The listing builds one solid part. Answer for the finished solid, in the listing's coordinates (mm). A direction names the side the tool comes from. Coordinates: 2 decimals unless noted, no trailing zeros. Loops run counter-clockwise (first coordinate to the right, second up) from the corner with the lowest first, then second, coordinate; pieces in that order, holes last. Notation, with made-up numbers: M 62.25,71 L 80.25,71 A20 cw 80.25,80 Z; hole C 7,52 d5. An arc over 180 degrees is marked long. Return JSON: item names as keys, results as strings. Group by question number.
1. Straight lines are drawn through the part: L1, parallel to Z at x = 30, y = -10; L2, parallel to X at y = -5.75, z = 19; L3, parallel to X at y = 10.25, z = 1.95. For each, find the intervals that lie inside material, in ascending order. Write a range as from..to.
2. Section C-C (y = 5) is taken. Count the separate pieces of the cut face and the enclosed holes in it, then the cut area to 3 significant figures.
3. Section D-D (x = -19) is taken. Write down the section's boundary in (y, z), then the cut area to 3 significant figures.
4. Given P1, Ø4.5, axis at x = -30, z = 11, coming from the +Y side; P2, Ø1.6, axis at x = -24, z = 11, coming from the +Y side; P3, Ø12, axis at x = -9, y = -14.5, coming from the +Z side, each flat-ended and moving along its own axis, determine where each tip first touches the part or whether it passes through.
5. Section B-B (z = 14.75) is taken. Write down the section's boundary in (x, y), then the cut area to 3 significant figures.
6. The mould has two halves that part along Y. Classify faces 6 (the face through (-10.32, 17.07, 2.54)), 7 (the face through (-22.8, -5.93, 11.62)), 8 (the face through (-27, 6.75, 14)): pulls with the +Y half, pulls with the -Y half, needs draft (parallel to the pull), parting line crosses it, or undercut.
7. Section A-A (y = 10.25) is taken. Write down the section's boundary in (x, z), then the cut area to 4 significant figures.
8. Which of the six approach directions +Z, -Z, +X, -X, +Y, -Y give full straight-line access (tool end or side, diameter ignored) to faces 1 (the face through (-20, -9, 14)), 2 (the face through (11.68, 17.07, 2.54)), 3 (the face through (-28.8, -5.93, 19.62)), 4 (the face through (0, -5, 0)), 5 (the face through (27, 6.75, 14))?
Autodesk Inventor part; units mm, degrees
ref_plane "YZ Plane" through (0, 0, 0) normal (1, 0, 0) x (0, 1, 0)
ref_plane "XZ Plane" through (0, 0, 0) normal (0, 1, 0) x (-1, 0, 0)
ref_plane "XY Plane" through (0, 0, 0) normal (0, 0, 1) x (1, 0, 0)
sketch "Sketch1" plane through (0, 0, 0) normal (0, 0, 1) x (1, 0, 0)
  line L0 (0, 0) -> (36, 0)
  line L1 (36, 0) -> (36, 25)
  line L2 (36, 25) -> (-36, 25)
  line L3 (-36, 25) -> (-36, -25)
  line L4 (-36, -25) -> (36, -25)
  line L5 (36, -25) -> (36, 25)
  dimension "d0" = 36
  dimension "d1" = 25
  dimension "d2" = 72
  dimension "d3" = 50
extrude "Extrusion1" add sketch "Sketch1" along normal blind 5
sketch "Sketch2" plane through (0, 0, 5) normal (0, 0, 1) x (1, 0, 0)
  line L0 (0, 0) -> (0, -25)
  line L1 (-36, -25) -> (36, -25)
  line L2 (0, -25) -> (0, 10.25)
  circle A0 centre (0, 10.25) radius 11.25
  dimension "d6" = 35.25
  dimension "d7" = 22.5
extrude "Extrusion2" cut sketch "Sketch2" against normal blind 22.5
sketch "Sketch3" plane through (0, 0, 5) normal (0, 0, 1) x (1, 0, 0)
  line L0 (0, 0) -> (11, 0)
  line L1 (11, -24.8696) -> (11, -21.6196)
  circle A0 centre (11, -21.6196) radius 1.475
  line L2 (0, 0) -> (0, -3.6992)
  circle A1 centre (-11, -21.6196) radius 1.475
  line L3 (11, -21.6196) -> (11, 18.3804)
  line L4 (11, -21.6196) -> (11, -1.6196)
  line L5 (11, -1.6196) -> (-3.4092, -1.6196)
  circle A2 centre (11, 18.3804) radius 1.475
  circle A3 centre (-11, 18.3804) radius 1.475
  point P0 (0, -1.6196)
  point P1 (11, -20.1446)
  point P2 (11, -23.0946)
  dimension "d10" = 11
  dimension "d11" = 3.25
  dimension "d12" = 2.95
  dimension "d15" = 40
  dimension "d16" = 20
extrude "Extrusion3" cut sketch "Sketch3" against normal blind 5 contours A0 L1 L3 | L3 L1 A0 | A1
sketch "Sketch4" plane through (0, 0, 5) normal (0, 0, 1) x (1, 0, 0)
  point P0 (0, 0)
extrude "Extrusion4" cut sketch "Sketch3" against normal blind 5 contours A2 | A3
sketch "Sketch5" plane through (36, -25, 0) normal (1, 0, 0) x (0, 0, -1)
  line L0 (0, 0) -> (0, 50)
  line L1 (-5, 0) -> (-5, 50)
  line L2 (0, 0) -> (-5, 0)
  line L3 (-5, 0) -> (-5, 50)
  line L4 (-5, 50) -> (0, 50)
  line L5 (0, 50) -> (0, 0)
  point P0 (0, 25)
  dimension "d19" = 5
ref_plane "Work Plane1" through (0, -25, 0) normal (1, 0, 0) x (0, 0, -1)
extrude "Extrusion5" cut sketch "Sketch5" against normal blind 1.5
mirror "Mirror1" about plane through (0, -25, 0) normal (1, 0, 0) of "Extrusion5"
sketch "Sketch6" plane through (34.5, -25, 0) normal (1, 0, 0) x (0, 0, -1)
  line L0 (-5, 0) -> (0, 0)
  line L1 (-5, 0) -> (-23, 0)
  line L2 (-23, 0) -> (-23, 34.75)
  line L3 (-23, 34.75) -> (-5, 34.75)
  line L4 (-5, 50) -> (-5, 0)
  line L5 (-5, 34.75) -> (-5, 0)
  point P0 (0, 25)
  dimension "d22" = 18
  dimension "d23" = 34.75
  dimension "d24" = 18
extrude "Extrusion6" add sketch "Sketch6" against normal blind 14.5
mirror "Mirror2" about plane through (0, -25, 0) normal (1, 0, 0) of "Extrusion6"
sketch "Sketch7" plane through (34.5, 9.75, 23) normal (0, 1, 0) x (1, 0, 0)
  line L0 (0, 0) -> (-14.5, 0)
  line L1 (0, 18) -> (0, 23)
  line L2 (0, 0) -> (0, 18)
  line L3 (0, 18) -> (0, 4)
  line L4 (0, 23) -> (0, 0)
  point P0 (-34.5, 23)
  point P1 (-10.5, 4)
  point P2 (-4.5, 4)
hole "Hole1" at (24, 9.75, 19) at (30, 9.75, 19) direction (0, -1, 0) diameter 2.7 depth 28 tip angle 118
mirror "Mirror3" about plane through (0, -25, 0) normal (1, 0, 0) of "Hole1"
sketch "Sketch8" plane through (34.5, 9.75, 23) normal (0, 1, 0) x (1, 0, 0)
  line L0 (0, 23) -> (0, 0)
  line L1 (0, 0) -> (0, 4)
  line L2 (0, 4) -> (-4.5, 4)
  line L3 (-4.5, 4) -> (-4.5, 12)
  line L4 (-4.5, 12) -> (-10.5, 12)
  point P0 (-34.5, 23)
  dimension "d45" = 4
  dimension "d46" = 4.5
  dimension "d47" = 8
  dimension "d48" = 6
hole "Hole2" at (24, 9.75, 11) at (30, 9.75, 11) direction (0, -1, 0) diameter 2.7 depth 28 tip angle 118
mirror "Mirror4" about plane through (0, -25, 0) normal (1, 0, 0) of "Hole2"
sketch "Sketch9" plane through (-34.5, 9.75, 23) normal (0, 1, 0) x (1, 0, 0)
  line L0 (0, 0) -> (14.5, 0)
  line L1 (0, 0) -> (74.2049, 0)
  line L2 (74.2049, 0) -> (74.2049, 18)
  line L3 (74.2049, 18) -> (0, 18)
  line L4 (0, 18) -> (0, 0)
  point P0 (34.5, 23)
extrude "Extrusion7" cut sketch "Sketch9" against normal blind 3
ref_plane "Work Plane2" through (0, -25, 0) normal (1, 0, 0) x (0, 0, -1)
equation "\"d8\" = d7"
properties part number "Front_plate"
Worked out:
{
 "1": {"L1": "0..9.65, 12.35..17.65, 20.35..23", "L2": "-34.5..-31.35, -28.65..-25.35, -22.65..-20, 20..22.65, 25.35..28.65, 31.35..34.5", "L3": "-34.5..-11.25, 11.25..34.5"},
 "2": {"separate pieces": "2", "enclosed holes": "8", "area": "722 mm^2"},
 "3": {"outline": "M -25,0 L 25,0 L 25,5 L -25,5 Z", "area": "250 mm^2"},
 "4": {"P1": "y = 6.75", "P2": "y = -18.58", "P3": "z = 5"},
 "5": {"outline": "M -34.5,-25 L -20,-25 L -20,6.75 L -34.5,6.75 Z; M 20,-25 L 34.5,-25 L 34.5,6.75 L 20,6.75 Z", "area": "921 mm^2"},
 "6": {"face 6": "undercut", "face 7": "needs draft", "face 8": "pulls with the +Y half"},
 "7": {"outline": "M -34.5,0 L -11.25,0 L -11.25,5 L -34.5,5 Z; M 11.25,0 L 34.5,0 L 34.5,5 L 11.25,5 Z", "area": "232.5 mm^2"},
 "8": {"face 1": "+Z, +Y, -Y", "face 2": "+Z, -Z", "face 3": "+Y", "face 4": "-Z, +X, -X, +Y, -Y", "face 5": "+Z, +X, -X, +Y"}
}
